Here's how the part is built. I have some questions about the finished solid (model axes, mm). A direction names the side the tool comes from. Coordinates: 2 decimals unless noted, no trailing zeros. Use a Markdown table: item, result.
```python
from build123d import *

# Parameters (mm, degrees)
F2_R     = 3.5
F3_DEPTH = 9.001
F4_R     = 5.75
F5_DEPTH = 8


with BuildPart() as f1:
    # F0 (on Front) → F1 (revolve)
    with BuildSketch(Plane.XZ):
        Polygon((0, 9), (0, 0), (51, 0), (51, 1), (49, 1), (49, 2), (47, 2), (47, 3), (45, 3), (45, 4), (43, 4), (43, 5), (41, 5), (41, 6), (39, 6), (39, 7), (37, 7), (37, 8), (35, 8), (35, 9), align=None)
    revolve(axis=Axis((0, 0, 4.5), (0, 0, 1)))

    # F2 (on face) → F3 (cut, through all)
    with BuildSketch(Plane.XY.offset(9)):
        Circle(F2_R)
    extrude(amount=-F3_DEPTH, mode=Mode.SUBTRACT)

    # F4 (on face) → F5 (cut)
    with BuildSketch(Plane(origin=(0, 0, 0), x_dir=(1, 0, 0), z_dir=(0, 0, -1))):
        Circle(F4_R)
    extrude(amount=-F5_DEPTH, mode=Mode.SUBTRACT)


solid = f1.part
```
1. We'd pull the mould along X, two halves only. Please class faces 1 (the face through (40, -25, 2)), 2 (the face through (-5.077, 38.668, 6.507)), 3 (the face through (-0.75, -5.7, 3.94)), 4 (the face through (3.233, -1.341, 8.507)): +X half, -X half, draft (parallel to the pull), parting line (faces both ways), or undercut.
Answers follow:
| item | result |
|---|---|
| face 1 | draft |
| face 2 | parting line |
| face 3 | undercut |
| face 4 | undercut |
2. Will these pins go through, and if not, where does the flat tip stop? pin 1 Ø8 at (x, y) = (0, 0) entering from -Z; pin 2 Ø4 at (x, z) = (19, 1) entering from +Y.
Answers follow:
| item | result |
|---|---|
| pin 1 | stops at z = 8 |
| pin 2 | stops at y = 48.08 |
3. Which directions (+Z, -Z, +X, -X, +Y, -Y) give clear straight access to the entire face, cutting with the end or side of a thin tool? Please do faces 5 (the face through (-11.056, -49.787, 0.507)), 6 (the face through (23.1, -36.5, 4)).
Answers follow:
| item | result |
|---|---|
| face 5 | +Z, -Z |
| face 6 | +Z |
4. I need wall thicknesses on probe 1 along Y at (x, z) = (0, 5.5); probe 2 along Y at (x, z) = (0, 8.8); probe 3 along Z at (x, y) = (-22.5, -42). Which ranges of each line are inside material? Lowest first, please.
Answers follow:
| item | result |
|---|---|
| probe 1 | y = -41 to -5.75, 5.75 to 41 |
| probe 2 | y = -35 to -3.5, 3.5 to 35 |
| probe 3 | z = 0 to 2 |
